Answer from the drawing. Dimensions are ordinates in mm from the lowest x, y and z of the part. Round coordinates to 2 decimals unless told otherwise and drop trailing zeros. Loops run counter-clockwise (first coordinate to the right, second up) from the corner with the lowest first, then second, coordinate; pieces in that order, holes last. Notation, with made-up numbers: M 75,5.25 L 117,5.25 A17 ccw 117,25.25 Z; hole C -22.75,38.25 d1. An arc over 180 degrees is marked long. One line per item, written item: value.
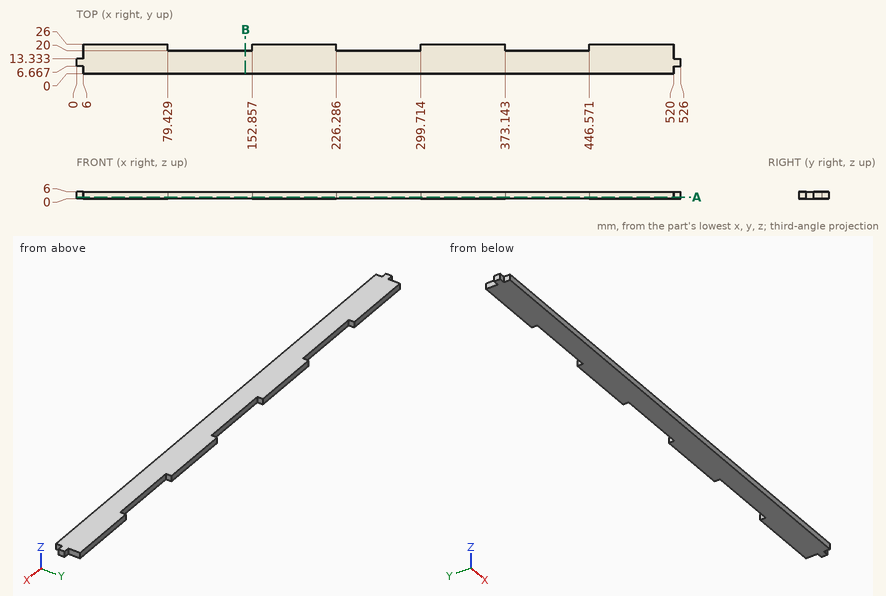
1) Find the intervals of material crossed by probe 1 along X at (y, z) = (21.75, 0.65) (1 decimal); probe 2 along Y at (x, z) = (237.5, 1.6); probe 3 along X at (y, z) = (17.75, 1.7), in increasing order. Write a range as from..to.
Check values:
probe 1: 6..79.4, 152.9..226.3, 299.7..373.1, 446.6..520
probe 2: 0..20
probe 3: 6..520
2) Each of these flat-tipped pins is pushed along its axis until it touches: pin 1 (3 mm diameter, centred on x = 322, z = 2, fed in from -Y); pin 2 (3 mm diameter, centred on x = 522.5, z = 4, fed in from +Y); pin 3 (1.8 mm diameter, centred on y = 23.5, z = 4, fed in from -X); pin 4 (1.8 mm diameter, centred on x = 522.5, z = 4, fed in from -Y). Where does it stop, or does it pass through?
Check values:
pin 1: y = 0
pin 2: y = 13.33
pin 3: x = 6
pin 4: y = 6.67
3) Find section A-A (z = 1.45). Give the vertices of the cut face in (x, y) (1 decimal).
Check values:
outline: M 0,6.7 L 6,6.7 L 6,0 L 520,0 L 520,6.7 L 526,6.7 L 526,13.3 L 520,13.3 L 520,26 L 446.6,26 L 446.6,20 L 373.1,20 L 373.1,26 L 299.7,26 L 299.7,20 L 226.3,20 L 226.3,26 L 152.9,26 L 152.9,20 L 79.4,20 L 79.4,26 L 6,26 L 6,13.3 L 0,13.3 Z
4) Find section B-B (x = 147). Give the vertices of the cut face in (y, z), then the cut area to 3 significant figures.
Check values:
outline: M 0,0 L 20,0 L 20,6 L 0,6 Z
area: 120 mm2
